Geometry: final body of the model. Coordinates: model frame, mm. Face numbers are marked on the shaded views. A direction names the side the tool comes from. Give positions to 0.01 mm unless a question says otherwise; leave off trailing zeros. Loops run counter-clockwise (first coordinate to the right, second up) from the corner with the lowest first, then second, coordinate; pieces in that order, holes last. Notation, with made-up numbers: (0.5, 79.5) - (24.5, 79.5) arc R19 ccw to (24.5, 91.5) - close; hole circle Ø7 at (89, -30.5). An arc over 180 degrees is marked (long way). Answer in a Markdown table with one row per item.
from build123d import *

# Parameters (mm, degrees)
F0_W           = 42
F0_H           = 15
F1_DEPTH       = 3.5
F2_W           = 42
F2_H           = 5
F3_DEPTH       = 1
F5_D           = 4.4
F5_CBORE_D     = 8.25
F5_CBORE_DEPTH = 4
F6_R           = 1.5
F7_DEPTH       = 15.001


with BuildPart() as f1:
    # F0 (on Top) → F1 (new body, symmetric)
    with BuildSketch(Plane.XY):
        Rectangle(F0_W, F0_H)
    extrude(amount=F1_DEPTH, both=True)

    # F2 (on face) → F3 (cut)
    with BuildSketch(Plane.XY.offset(3.5)):
        Rectangle(F2_W, F2_H)
    extrude(amount=-F3_DEPTH, mode=Mode.SUBTRACT)

    # F5 (through all)
    with Locations(Plane(origin=(0, 0, -3.5), x_dir=(1, 0, 0), z_dir=(0, 0, -1))):
        with Locations((9, 0), (-9, 0)):
            CounterBoreHole(F5_D / 2, F5_CBORE_D / 2, F5_CBORE_DEPTH)

    # F6 (on face) → F7 (cut, through all)
    with BuildSketch(Plane(origin=(0, 7.5, 0), x_dir=(-1, 0, 0), z_dir=(0, 1, 0))):
        with Locations((-13, 0)):
            Circle(F6_R)
        with Locations((13, 0)):
            Circle(F6_R)
    extrude(amount=-F7_DEPTH, mode=Mode.SUBTRACT)


solid = f1.part
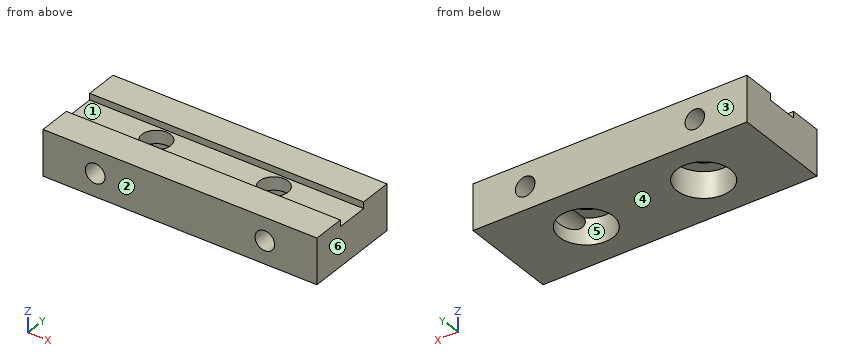
Q1. Reachability of the marked faces 5 and 6 from +Z, -Z, +X, -X, +Y, -Y: full face, straight path, thin tool, end or side. Return the list, or none.
Check values:
| item | result |
|---|---|
| face 5 | -Z |
| face 6 | +Z, -Z, +X, +Y, -Y |
Q2. Draft query along Y for the marked faces 1, 2, 3 and 4. Return one class per face: pulls with the +Y half, pulls with the -Y half, needs draft (parallel to the pull), parting line crosses it, or undercut.
Check values:
| item | result |
|---|---|
| face 1 | undercut |
| face 2 | pulls with the -Y half |
| face 3 | pulls with the +Y half |
| face 4 | needs draft |
Q3. Cut plane B-B (z = -2.25). Output: boundary loops of the cut face in (x, y) (3 decimals).
Check values:
| item | result |
|---|---|
| outline | (-21, -7.5) - (21, -7.5) - (21, 7.5) - (-21, 7.5) - close; hole circle Ø8.25 at (-9, 0); hole circle Ø8.25 at (9, 0) |
Q4. Cut plane C-C (y = -5.25). Output: boundary loops of the cut face in (x, z), and give its area (3 significant figures).
Check values:
| item | result |
|---|---|
| outline | (-21, -3.5) - (21, -3.5) - (21, 3.5) - (-21, 3.5) - close; hole circle Ø3 at (-13, 0); hole circle Ø3 at (13, 0) |
| area | 280 mm² |
Q5. Cut plane D-D (x = -3). Output: boundary loops of the cut face in (y, z).
Check values:
| item | result |
|---|---|
| outline | (-7.5, -3.5) - (7.5, -3.5) - (7.5, 3.5) - (2.5, 3.5) - (2.5, 2.5) - (-2.5, 2.5) - (-2.5, 3.5) - (-7.5, 3.5) - close |
Q6. Cut plane A-A (x = -9). Output: boundary loops of the cut face in (y, z) (3 decimals), and give its area (3 significant figures).
Check values:
| item | result |
|---|---|
| outline | (-7.5, -3.5) - (-4.125, -3.5) - (-4.125, 0.5) - (-2.2, 0.5) - (-2.2, 2.5) - (-2.5, 2.5) - (-2.5, 3.5) - (-7.5, 3.5) - close; (2.2, 0.5) - (4.125, 0.5) - (4.125, -3.5) - (7.5, -3.5) - (7.5, 3.5) - (2.5, 3.5) - (2.5, 2.5) - (2.2, 2.5) - close |
| area | 58.2 mm² |
Q7. First-contact query: pin 1 (3.5 mm diameter, centred on x = -13, z = 0, fed in from -Y); pin 2 (7 mm diameter, centred on x = 9, y = 0, fed in from -Z); pin 3 (3.5 mm diameter, centred on x = -9, y = 0, fed in from +Z); pin 4 (1.5 mm diameter, centred on x = 12, y = 1.5, fed in from +Z). Flat tips, straight axial feed; report the tip coordinate or a pass-through.
Check values:
| item | result |
|---|---|
| pin 1 | y = -7.5 |
| pin 2 | z = 0.5 |
| pin 3 | through |
| pin 4 | z = 2.5 |
Q8. Material intervals for line 1 along X through (y, z) = (-0.25, -2); line 2 along Z through (x, y) = (-13, 4); line 3 along Y through (x, z) = (-9, 1.5), sorted ascending.
Check values:
| item | result |
|---|---|
| line 1 | -21 to -13.12, -4.88 to 4.88, 13.12 to 21 |
| line 2 | -3.5 to -1.5, 1.5 to 3.5 |
| line 3 | -7.5 to -2.2, 2.2 to 7.5 |
